from build123d import *

# Parameters (mm, degrees)
F0_W      = 38.1
F0_H      = 76.2
F1_DEPTH  = 12.7
F2_R      = 9.525
F3_DEPTH  = 38.1
F4_R      = 6.35
F5_DEPTH  = 40.386
F6_W      = 482.6
F6_H      = 292.1
F7_DEPTH  = 13.716
F8_R      = 5.08
F10_DEPTH = 0.254


with BuildPart() as f1:
    # F0 (on Front) → F1 (new body)
    with BuildSketch(Plane.XZ):
        Rectangle(F0_W, F0_H)
    extrude(amount=F1_DEPTH)

    # F2 (on face) → F3 (join)
    with BuildSketch(Plane.YZ.offset(19.05)):
        with Locations((-12.7, 0)):
            Circle(F2_R)
    extrude(amount=-F3_DEPTH)

    # F4 (on face) → F5 (cut)
    with BuildSketch(Plane.YZ.offset(19.05)):
        with Locations((-12.7, 0)):
            Circle(F4_R)
    extrude(amount=-F5_DEPTH, mode=Mode.SUBTRACT)

    # F6 (on face) → F7 (join)
    with BuildSketch(Plane(origin=(0, 0, 0), x_dir=(-1, 0, 0), z_dir=(0, 1, 0))):
        Rectangle(F6_W, F6_H)
    extrude(amount=F7_DEPTH)

    # F8
    f8_edges = [f1.edges().sort_by_distance(p)[0] for p in [
        (-241.3, 6.858, 146.05),
        (-241.3, 6.858, -146.05),
        (241.3, 6.858, -146.05),
        (241.3, 6.858, 146.05),
        (241.3, 0, 0),
        (0, 0, 146.05),
        (-241.3, 0, 0),
        (0, 0, -146.05),
    ]]
    fillet(f8_edges, radius=F8_R)

    # F9 (on face) → F10 (cut)
    with BuildSketch(Plane(origin=(0, 13.716, 0), x_dir=(-1, 0, 0), z_dir=(0, 1, 0))):
        with BuildLine():
            Line((-234.569, -139.7), (234.569, -139.7))
            ThreePointArc((234.569, -139.7), (234.838408, -139.588408), (234.95, -139.319))
            Line((234.95, -139.319), (234.95, 139.319))
            ThreePointArc((234.95, 139.319), (234.838408, 139.588408), (234.569, 139.7))
            Line((234.569, 139.7), (-234.569, 139.7))
            ThreePointArc((-234.569, 139.7), (-234.838408, 139.588408), (-234.95, 139.319))
            Line((-234.95, 139.319), (-234.95, -139.319))
            ThreePointArc((-234.95, -139.319), (-234.838408, -139.588408), (-234.569, -139.7))
        make_face()
    extrude(amount=-F10_DEPTH, mode=Mode.SUBTRACT)


solid = f1.part
Work out the finished part from the listing and answer in its coordinate system (mm). A direction names the side the tool comes from. Round coordinates to 2 decimals unless told otherwise and drop trailing zeros. Write each loop counter-clockwise with the first axis right and the second up, starting at its lowest first coordinate (ties: lowest second). Pieces come first, ordered by that corner, then holes. Notation, with made-up numbers: (40.5, -26.5) - (94.5, -26.5) arc R23 cw to (94.5, 11.5) - close; hole circle Ø2 at (55, -8.5). An arc over 180 degrees is marked (long way). Answer in a Markdown table with one row per item. Add a question column.
1. For faces 1 (the flat face through (0, -12.7, 24)), 2 (the flat face through (0, -6, -38.1)), 3 (the flat face through (19.05, -6, -1)), 4 (the flat face through (-19.05, -6, -1)), determine the directions among +Z, -Z, +X, -X, +Y, -Y from which every point of the face is accessible in a straight line to the end or side of a thin tool.
2. A cutting plane is placed at A-A, the plane z = 0. Determine the outline of the cut face in (x, y) (3 decimals).
3. A cutting plane is placed at B-B, the plane x = 14.5. Determine the outline of the cut face in (y, z) (3 decimals).
4. Given pin 1 (14 mm diameter, centred on x = 0, y = -3.5, fed in from +Z); pin 2 (7.5 mm diameter, centred on y = -12.7, z = 0, fed in from +X); pin 3 (4 mm diameter, centred on y = -1.5, z = -26.5, fed in from +X); pin 4 (23 mm diameter, centred on x = -8, z = 17, fed in from -Y), each flat-ended and moving along its own axis, determine where each tip first touches the part or whether it passes through.
5. The mould has two halves that part along Y. Classify faces 5 (the cylindrical face through (0.267, -6.643, 1.907)), 6 (the cylindrical face through (0.267, -22.223, 0.209)), 7 (the flat face through (3, 9, -146.05)): +Y half, -Y half, draft (parallel to the pull), parting line (faces both ways), or undercut.
6. Find the intervals of material crossed by line 1 along Z through (x, y) = (-1, -12); line 2 along Y through (x, z) = (-70, -32); line 3 along X through (y, z) = (-6, 19), in increasing order. Write a range as from..to.
7. A cutting plane is placed at C-C, the plane z = 114. Determine the outline of the cut face in (x, y).
Worked out:
| question | item | result |
|---|---|---|
| 1 | face 1 | +Z, +X, -X, -Y |
| 1 | face 2 | -Z, +X, -X, -Y |
| 1 | face 3 | +Z, -Z, +X, -Y |
| 1 | face 4 | +Z, -Z, -X, -Y |
| 2 | outline | (-241.3, 5.08) arc R5.08 ccw to (-236.22, 0) - (-19.05, 0) - (-19.05, -6.35) - (19.05, -6.35) - (19.05, 0) - (236.22, 0) arc R5.08 ccw to (241.3, 5.08) - (241.3, 13.716) - (234.95, 13.716) - (234.95, 13.462) - (-234.95, 13.462) - (-234.95, 13.716) - (-241.3, 13.716) - close; (-19.05, -22.225) - (19.05, -22.225) - (19.05, -19.05) - (-19.05, -19.05) - close |
| 3 | outline | (-12.7, -38.1) - (0, -38.1) - (0, -140.97) arc R5.08 ccw to (5.08, -146.05) - (13.716, -146.05) - (13.716, -139.7) - (13.462, -139.7) - (13.462, 139.7) - (13.716, 139.7) - (13.716, 146.05) - (5.08, 146.05) arc R5.08 ccw to (0, 140.97) - (0, 38.1) - (-12.7, 38.1) - (-12.7, 9.525) arc R9.525 ccw to (-12.7, -9.525) - close; hole circle Ø12.7 at (-12.7, 0) |
| 4 | pin 1 | z = 145.8 |
| 4 | pin 2 | through |
| 4 | pin 3 | x = 238.42 |
| 4 | pin 4 | y = -20.48 |
| 5 | face 5 | undercut |
| 5 | face 6 | -Y half |
| 5 | face 7 | draft |
| 6 | line 1 | -38.1..-6.31, 6.31..38.1 |
| 6 | line 2 | 0..13.46 |
| 6 | line 3 | -19.05..19.05 |
| 7 | outline | (-241.3, 5.08) arc R5.08 ccw to (-236.22, 0) - (236.22, 0) arc R5.08 ccw to (241.3, 5.08) - (241.3, 13.72) - (234.95, 13.72) - (234.95, 13.46) - (-234.95, 13.46) - (-234.95, 13.72) - (-241.3, 13.72) - close |
